Here's how the part is built. I have some questions about the finished solid (model axes, mm). Face numbers are marked on the shaded views. A direction names the side the tool comes from. Round coordinates to 2 decimals unless told otherwise and drop trailing zeros. Order: outer loops, then holes, each group sorted by start corner. A loop starts at its lowest first (then second) coordinate and runs counter-clockwise, first axis right, second up. Notation, with made-up numbers: (73.5, -17.5) -> (77.5, -17.5) arc R32 cw to (77.5, 20.5) -> close; hole circle Ø10 at (-24, 47). An arc over 180 degrees is marked (long way). Answer in a Markdown table with one row per item.
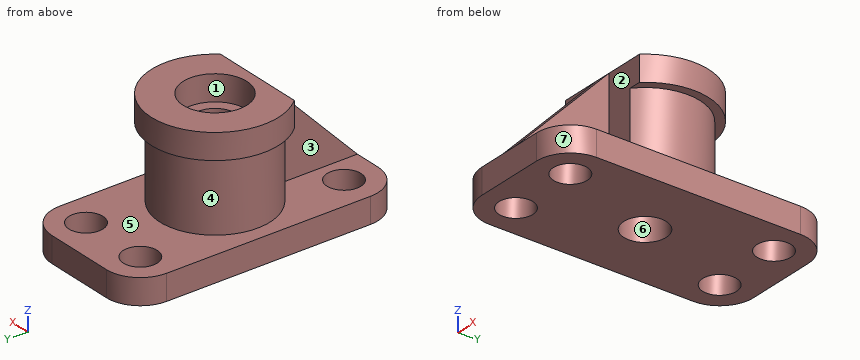
```python
from build123d import *

# Parameters (mm, degrees)
IZIM1_R                     = 8
Y_KSEKLIK_EKSTR_ZYON2_DEPTH = 12
IZIM2_R                     = 26
IZIM2_R_2                   = 10
Y_KSEKLIK_EKSTR_ZYON3_DEPTH = 34
KES_EKSTR_ZYON1_START       = -34
IZIM3_R                     = 10
KES_EKSTR_ZYON1_DEPTH       = 34
IZIM4_R                     = 30
IZIM4_R_2                   = 15
Y_KSEKLIK_EKSTR_ZYON4_DEPTH = 12
IZIM6_W                     = 47.489367516
IZIM6_H                     = 14.251313653
KES_EKSTR_ZYON2_DEPTH       = 46
FEDER1_REACH                = 120.683
IZIM9_WALL_W                = 303.022183262
IZIM9_WALL_H                = 8


with BuildPart() as part:
    # Çizim1 → Yükseklik-Ekstrüzyon2 (new body)
    with BuildSketch(Plane.XY):
        with BuildLine():
            Line((-85.16772712, 82.313308987), (-85.16772712, -13.686691013))
            ThreePointArc((-85.16772712, -13.686691013), (-80.481435619, -25.000399512), (-69.16772712, -29.686691013))
            Line((-69.16772712, -29.686691013), (-36.16772712, -29.686691013))
            ThreePointArc((-36.16772712, -29.686691013), (-24.854018621, -25.000399512), (-20.16772712, -13.686691013))
            Line((-20.16772712, -13.686691013), (-20.16772712, 82.313308987))
            ThreePointArc((-20.16772712, 82.313308987), (-24.854018621, 93.627017486), (-36.16772712, 98.313308987))
            Line((-36.16772712, 98.313308987), (-69.16772712, 98.313308987))
            ThreePointArc((-69.16772712, 98.313308987), (-80.481435619, 93.627017486), (-85.16772712, 82.313308987))
        make_face()
        with Locations((-69.16772712, 82.313308987)):
            Circle(IZIM1_R, mode=Mode.SUBTRACT)
        with Locations((-36.16772712, 82.313308987)):
            Circle(IZIM1_R, mode=Mode.SUBTRACT)
        with Locations((-69.16772712, -13.686691013)):
            Circle(IZIM1_R, mode=Mode.SUBTRACT)
        with Locations((-36.16772712, -13.686691013)):
            Circle(IZIM1_R, mode=Mode.SUBTRACT)
    extrude(amount=Y_KSEKLIK_EKSTR_ZYON2_DEPTH)

    # Çizim2 → Yükseklik-Ekstrüzyon3 (add)
    with BuildSketch(Plane.XY.offset(12)):
        with Locations((-52.66772712, 34.313308987)):
            Circle(IZIM2_R)
        with Locations((-52.66772712, 34.313308987)):
            Circle(IZIM2_R_2, mode=Mode.SUBTRACT)
    extrude(amount=Y_KSEKLIK_EKSTR_ZYON3_DEPTH)

    # Çizim3 → Kes-Ekstrüzyon1 (cut)
    with BuildSketch(Plane.XY.offset(12).offset(KES_EKSTR_ZYON1_START)):
        with Locations((-52.66772712, 34.313308987)):
            Circle(IZIM3_R)
    extrude(amount=KES_EKSTR_ZYON1_DEPTH, mode=Mode.SUBTRACT)

    # Çizim4 → Yükseklik-Ekstrüzyon4 (add)
    with BuildSketch(Plane.XY.offset(46)):
        with Locations((-52.66772712, 34.313308987)):
            Circle(IZIM4_R)
        with Locations((-52.66772712, 34.313308987)):
            Circle(IZIM4_R_2, mode=Mode.SUBTRACT)
    extrude(amount=Y_KSEKLIK_EKSTR_ZYON4_DEPTH)

    # Çizim6 → Kes-Ekstrüzyon2 (cut)
    with BuildSketch(Plane.XY.offset(58)):
        with Locations((-51.283723137, 7.187652161)):
            Rectangle(IZIM6_W, IZIM6_H)
    extrude(amount=-KES_EKSTR_ZYON2_DEPTH, mode=Mode.SUBTRACT)

    # Çizim9 wall → Feder1 (add, up to next)
    with BuildSketch(Plane(origin=(-52.66772712, -7.686691013, 35), x_dir=(0, -0.691222645967, -0.722641857148), z_dir=(0, -0.722641857148, 0.691222645967)), mode=Mode.PRIVATE) as feder1_sk1:
        Rectangle(IZIM9_WALL_W, IZIM9_WALL_H)
    feder1_tool1 = extrude(feder1_sk1.sketch, amount=-FEDER1_REACH, mode=Mode.PRIVATE) - part.part
    add(feder1_tool1.solids().sort_by_distance((-52.66772712, -7.686691013, 35))[0])


solid = part.part
```
1. Suppose I cut it at D-D on x = -72. Write out the boundary of the cut face in (y, z).
Numbers:
| item | result |
|---|---|
| outline | (-29.43, 0) -> (-21.17, 0) -> (-21.17, 12) -> (-29.43, 12) -> close; (-6.2, 0) -> (74.83, 0) -> (74.83, 12) -> (51.7, 12) -> (51.7, 46) -> (57.25, 46) -> (57.25, 58) -> (14.31, 58) -> (14.31, 46) -> (16.93, 46) -> (16.93, 12) -> (-6.2, 12) -> close; (89.8, 0) -> (98.06, 0) -> (98.06, 12) -> (89.8, 12) -> close |
2. Suppose I cut it at A-A on y = 29. Write out the boundary of the cut face in (x, z), then the cut area to 3 significant figures.
Numbers:
| item | result |
|---|---|
| outline | (-85.17, 0) -> (-61.14, 0) -> (-61.14, 46) -> (-66.7, 46) -> (-66.7, 58) -> (-82.19, 58) -> (-82.19, 46) -> (-78.12, 46) -> (-78.12, 12) -> (-85.17, 12) -> close; (-44.2, 0) -> (-20.17, 0) -> (-20.17, 12) -> (-27.22, 12) -> (-27.22, 46) -> (-23.14, 46) -> (-23.14, 58) -> (-38.64, 58) -> (-38.64, 46) -> (-44.2, 46) -> close |
| area | 2,100 mm2 |
3. We'd pull the mould along X, two halves only. Please class the marked faces 5, 6 and 7: released by +X, released by -X, zero draft, split by the parting line, or undercut.
Numbers:
| item | result |
|---|---|
| face 5 | zero draft |
| face 6 | undercut |
| face 7 | released by +X |
4. For pin 1 Ø2 at (x, y) = (-29, 64) entering from +Z; pin 2 Ø25 at (x, y) = (-41, 27.5) entering from -Z; pin 3 Ø15 at (x, y) = (-53, 28.5) entering from +Z; pin 4 Ø22 at (y, z) = (-11.5, 35.5) entering from -X, each with a flat end and sliding along its axis, tell me the tip position at first contact or that it passes through.
Numbers:
| item | result |
|---|---|
| pin 1 | stops at z = 12 |
| pin 2 | stops at z = 0 |
| pin 3 | stops at z = 46 |
| pin 4 | stops at x = -56.67 |
5. For the marked faces 1, 2, 3 and 4, which set-ups out of +Z, -Z, +X, -X, +Y, -Y let a thin tool reach every point of the face, with its end or its side?
Numbers:
| item | result |
|---|---|
| face 1 | +Z |
| face 2 | +Z, +X, -Y |
| face 3 | +Z, -X, -Y |
| face 4 | none |
6. Suppose I cut it at B-B on z = 17. Write out the boundary of the cut face in (x, y).
Numbers:
| item | result |
|---|---|
| outline | (-69.28, 14.31) -> (-56.67, 14.31) -> (-56.67, -24.9) -> (-48.67, -24.9) -> (-48.67, 14.31) -> (-36.05, 14.31) arc R26 ccw (long way) to start; hole circle Ø20 at (-52.67, 34.31) |
7. Please list where these lines run through material, in increasing order: line 1 along Z through (x, y) = (-27, 23.5); line 2 along X through (y, z) = (79.5, 8); line 3 along Z through (x, y) = (-60, -12).
Numbers:
| item | result |
|---|---|
| line 1 | z = 0 to 12, 46 to 58 |
| line 2 | x = -85.17 to -76.66, -61.68 to -43.66, -28.68 to -20.17 |
| line 3 | z = 0 to 12 |
8. Suppose I cut it at C-C on x = -25. Write out the boundary of the cut face in (y, z).
Numbers:
| item | result |
|---|---|
| outline | (-25.14, 0) -> (93.77, 0) -> (93.77, 12) -> (-25.14, 12) -> close; (22.72, 46) -> (45.91, 46) -> (45.91, 58) -> (22.72, 58) -> close |
